Read the model definition and answer for the solid it produces. Units are mm, in the model's axes. A direction names the side the tool comes from. Give positions to 0.01 mm unless a question says otherwise; leave off trailing zeros. Loops run counter-clockwise (first coordinate to the right, second up) from the corner with the lowest first, then second, coordinate; pieces in that order, holes last.
(1) Straight lines are drawn through the part: probe 1 along Y at (x, z) = (0.25, 14); probe 2 along Y at (x, z) = (-3, 10); probe 3 along X at (y, z) = (9, 4.5). For each, find the intervals that lie inside material, in ascending order.
(2) Which of the six approach directions +Z, -Z, +X, -X, +Y, -Y give full straight-line access (tool end or side, diameter ignored) to faces 4 (the face through (0, 15.5, 14)), 5 (the face through (0, 17.5, 7)), 6 (the face through (0, 16, 6))?
(3) Find section D-D, the plane x = 7. Write down the section's boundary in (y, z).
(4) Find section C-C, the plane z = -0.5. Write down the section's boundary in (x, y), then the cut area to 3 significant figures.
(5) Find section A-A, the plane x = 2.5. Write down the section's boundary in (y, z), then the cut area to 3 significant figures.
(6) Determine the mould class of faces 1 (the face through (-7.5, 0, 7)), 2 (the face through (-6, 0, 6)), 3 (the face through (7.5, 0, 7)) for opening direction X: pulls with the +X half, pulls with the -X half, needs draft (parallel to the pull), parting line crosses it, or undercut.
(7) Find section B-B, the plane y = 12.5. Write down the section's boundary in (x, z).
(8) Each of these flat-tipped pins is pushed along its axis until it touches: P1, Ø6, axis at x = -2, z = 6.5, coming from the +Y side; P2, Ø5, axis at x = -6, z = 10.5, coming from the -Y side; P3, Ø7.5, axis at y = 4, z = 5.5, coming from the +X side; P4, Ø13, axis at x = 2.5, y = -2, coming from the -Z side. Where does it stop, or does it pass through?
```python
from build123d import *

# Parameters (mm, degrees)
SKETCH1_W           = 15
SKETCH1_H           = 35
BOSS_EXTRUDE1_DEPTH = 15
SKETCH3_W           = 12
SKETCH3_H           = 32
CUT_EXTRUDE2_DEPTH  = 13.5
SKETCH4_W           = 23
SKETCH4_H           = 43
SKETCH4_W_2         = 12
SKETCH4_H_2         = 32
BOSS_EXTRUDE2_DEPTH = 2
SKETCH5_W           = 1
SKETCH5_H           = 31
CUT_EXTRUDE3_DEPTH  = 2


with BuildPart() as part:
    # Sketch1 → Boss-Extrude1 (new body)
    with BuildSketch(Plane.XY):
        Rectangle(SKETCH1_W, SKETCH1_H)
    extrude(amount=BOSS_EXTRUDE1_DEPTH)

    # Sketch3 → Cut-Extrude2 (cut)
    with BuildSketch(Plane(origin=(0, 0, 0), x_dir=(-1, 0, 0), z_dir=(0, 0, -1))):
        Rectangle(SKETCH3_W, SKETCH3_H)
    extrude(amount=-CUT_EXTRUDE2_DEPTH, mode=Mode.SUBTRACT)

    # Sketch4 → Boss-Extrude2 (add)
    with BuildSketch(Plane(origin=(0, 0, 0), x_dir=(-1, 0, 0), z_dir=(0, 0, -1))):
        Rectangle(SKETCH4_W, SKETCH4_H)
        Rectangle(SKETCH4_W_2, SKETCH4_H_2, mode=Mode.SUBTRACT)
    extrude(amount=BOSS_EXTRUDE2_DEPTH)

    # Sketch5 → Cut-Extrude3 (cut)
    with BuildSketch(Plane.XY.offset(15)):
        Rectangle(SKETCH5_W, SKETCH5_H)
    extrude(amount=-CUT_EXTRUDE3_DEPTH, mode=Mode.SUBTRACT)


solid = part.part
```
Entries:
1. probe 1: y = -17.5 to -15.5, 15.5 to 17.5
1. probe 2: y = -17.5 to -16, 16 to 17.5
1. probe 3: x = -7.5 to -6, 6 to 7.5
2. face 4: +Z, -Z
2. face 5: +Z, +X, -X, +Y
2. face 6: -Z
3. outline: (-21.5, -2) - (21.5, -2) - (21.5, 0) - (17.5, 0) - (17.5, 15) - (-17.5, 15) - (-17.5, 0) - (-21.5, 0) - close
4. outline: (-11.5, -21.5) - (11.5, -21.5) - (11.5, 21.5) - (-11.5, 21.5) - close; hole (-6, -16) - (6, -16) - (6, 16) - (-6, 16) - close
4. area: 605 mm2
5. outline: (-21.5, -2) - (-16, -2) - (-16, 13.5) - (16, 13.5) - (16, -2) - (21.5, -2) - (21.5, 0) - (17.5, 0) - (17.5, 15) - (-17.5, 15) - (-17.5, 0) - (-21.5, 0) - close
5. area: 115 mm2
6. face 1: pulls with the -X half
6. face 2: undercut
6. face 3: pulls with the +X half
7. outline: (-11.5, -2) - (-6, -2) - (-6, 13.5) - (-0.5, 13.5) - (-0.5, 15) - (-7.5, 15) - (-7.5, 0) - (-11.5, 0) - close; (0.5, 13.5) - (6, 13.5) - (6, -2) - (11.5, -2) - (11.5, 0) - (7.5, 0) - (7.5, 15) - (0.5, 15) - close
8. P1: stops at y = 17.5
8. P2: stops at y = -17.5
8. P3: stops at x = 7.5
8. P4: stops at z = -2
